```python
from build123d import *

# Parameters (mm, degrees)
SKETCH1_R           = 50
SKETCH1_W           = 25.4
SKETCH1_H           = 25.4
BOSS_EXTRUDE1_DEPTH = 5


with BuildPart() as part:
    # Sketch1 → Boss-Extrude1 (new body)
    with BuildSketch(Plane(origin=(0, 0, 0), x_dir=(1, 0, 0), z_dir=(0, 1, 0))):
        with BuildLine():
            Line((175.4, 110), (201.990098767, 110))
            ThreePointArc((201.990098767, 110), (230, 0), (201.990098767, -110))
            Line((201.990098767, -110), (175.4, -110))
            Line((175.4, -110), (175.4, -115))
            Line((175.4, -115), (199.18584287, -115))
            ThreePointArc((199.18584287, -115), (162.634559673, -162.634559673), (115, -199.18584287))
            Line((115, -199.18584287), (115, -175.4))
            Line((115, -175.4), (110, -175.4))
            Line((110, -175.4), (110, -201.990098767))
            ThreePointArc((110, -201.990098767), (0, -230), (-110, -201.990098767))
            Line((-110, -201.990098767), (-110, -175.4))
            Line((-110, -175.4), (-115, -175.4))
            Line((-115, -175.4), (-115, -199.18584287))
            ThreePointArc((-115, -199.18584287), (-162.634559673, -162.634559673), (-199.18584287, -115))
            Line((-199.18584287, -115), (-175.4, -115))
            Line((-175.4, -115), (-175.4, -110))
            Line((-175.4, -110), (-201.990098767, -110))
            ThreePointArc((-201.990098767, -110), (-230, 0), (-201.990098767, 110))
            Line((-201.990098767, 110), (-175.4, 110))
            Line((-175.4, 110), (-175.4, 115))
            Line((-175.4, 115), (-199.18584287, 115))
            ThreePointArc((-199.18584287, 115), (-162.634559673, 162.634559673), (-115, 199.18584287))
            Line((-115, 199.18584287), (-115, 175.4))
            Line((-115, 175.4), (-110, 175.4))
            Line((-110, 175.4), (-110, 201.990098767))
            ThreePointArc((-110, 201.990098767), (0, 230), (110, 201.990098767))
            Line((110, 201.990098767), (110, 175.4))
            Line((110, 175.4), (115, 175.4))
            Line((115, 175.4), (115, 199.18584287))
            ThreePointArc((115, 199.18584287), (162.634559673, 162.634559673), (199.18584287, 115))
            Line((199.18584287, 115), (175.4, 115))
            Line((175.4, 115), (175.4, 110))
        make_face()
        with Locations(Location((0, 0, 0), (0, 0, 270))):
            Circle(SKETCH1_R, mode=Mode.SUBTRACT)
        with Locations((127.7, 127.7)):
            Rectangle(SKETCH1_W, SKETCH1_H, mode=Mode.SUBTRACT)
        with Locations((-127.7, 127.7)):
            Rectangle(SKETCH1_W, SKETCH1_H, mode=Mode.SUBTRACT)
        with Locations((127.7, -127.7)):
            Rectangle(SKETCH1_W, SKETCH1_H, mode=Mode.SUBTRACT)
        with Locations((-127.7, -127.7)):
            Rectangle(SKETCH1_W, SKETCH1_H, mode=Mode.SUBTRACT)
        with BuildLine():
            Line((184.4, 26.5), (184.4, -26.5))
            ThreePointArc((184.4, -26.5), (183.374873734, -28.974873734), (180.9, -30))
            Line((180.9, -30), (179.9, -30))
            ThreePointArc((179.9, -30), (177.425126266, -28.974873734), (176.4, -26.5))
            Line((176.4, -26.5), (176.4, 26.5))
            ThreePointArc((176.4, 26.5), (177.425126266, 28.974873734), (179.9, 30))
            Line((179.9, 30), (180.9, 30))
            ThreePointArc((180.9, 30), (183.374873734, 28.974873734), (184.4, 26.5))
        make_face(mode=Mode.SUBTRACT)
        with BuildLine():
            Line((-26.5, 184.4), (26.5, 184.4))
            ThreePointArc((26.5, 184.4), (28.974873734, 183.374873734), (30, 180.9))
            Line((30, 180.9), (30, 179.9))
            ThreePointArc((30, 179.9), (28.974873734, 177.425126266), (26.5, 176.4))
            Line((26.5, 176.4), (-26.5, 176.4))
            ThreePointArc((-26.5, 176.4), (-28.974873734, 177.425126266), (-30, 179.9))
            Line((-30, 179.9), (-30, 180.9))
            ThreePointArc((-30, 180.9), (-28.974873734, 183.374873734), (-26.5, 184.4))
        make_face(mode=Mode.SUBTRACT)
        with BuildLine():
            Line((26.5, -184.4), (-26.5, -184.4))
            ThreePointArc((-26.5, -184.4), (-28.974873734, -183.374873734), (-30, -180.9))
            Line((-30, -180.9), (-30, -179.9))
            ThreePointArc((-30, -179.9), (-28.974873734, -177.425126266), (-26.5, -176.4))
            Line((-26.5, -176.4), (26.5, -176.4))
            ThreePointArc((26.5, -176.4), (28.974873734, -177.425126266), (30, -179.9))
            Line((30, -179.9), (30, -180.9))
            ThreePointArc((30, -180.9), (28.974873734, -183.374873734), (26.5, -184.4))
        make_face(mode=Mode.SUBTRACT)
        with BuildLine():
            Line((-184.4, -26.5), (-184.4, 26.5))
            ThreePointArc((-184.4, 26.5), (-183.374873734, 28.974873734), (-180.9, 30))
            Line((-180.9, 30), (-179.9, 30))
            ThreePointArc((-179.9, 30), (-177.425126266, 28.974873734), (-176.4, 26.5))
            Line((-176.4, 26.5), (-176.4, -26.5))
            ThreePointArc((-176.4, -26.5), (-177.425126266, -28.974873734), (-179.9, -30))
            Line((-179.9, -30), (-180.9, -30))
            ThreePointArc((-180.9, -30), (-183.374873734, -28.974873734), (-184.4, -26.5))
        make_face(mode=Mode.SUBTRACT)
    extrude(amount=BOSS_EXTRUDE1_DEPTH)


solid = part.part
```
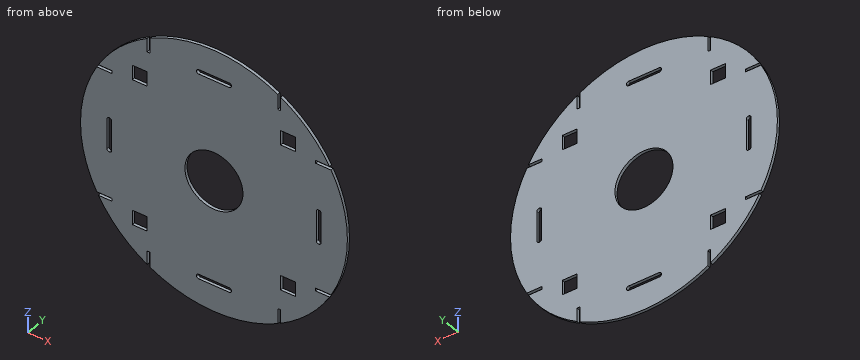
Input: part model. Units: mm. Frame: model coordinates. Give positions to 0.01 mm unless a question says otherwise; leave off trailing zeros. Write each loop counter-clockwise with the first axis right and the second up, starting at its lowest first coordinate (ties: lowest second). Pieces come first, ordered by that corner, then holes. Notation, with made-up numbers: (65.5, 73.5) - (109.5, 73.5) arc R24 cw to (109.5, 86.5) - close; hole circle Ø11 at (60.25, 73). An arc over 180 degrees is marked (long way). Write item = value, one per line. Start each with the question number.
1. Section query A-A, the plane z = 0. Output: boundary loops of the cut face in (x, y).
2. Section query C-C, the plane z = 135. Output: boundary loops of the cut face in (x, y).
3. First-contact query: pin 1 Ø2.5 at (y, z) = (2.5, 134) entering from -X; pin 2 Ø3 at (y, z) = (4.5, 98) entering from -X; pin 3 Ø2.5 at (x, y) = (-127.5, 3.5) entering from +Z. Flat tips, straight axial feed; report the tip coordinate or a pass-through.
4. Ray query, L1, parallel to X at y = 4.55, z = -18; L2, parallel to X at y = 2.8, z = 121.5; L3, parallel to Z at x = 123.5, y = 0.8. Return the intervals inside material, ascending.
5. Section query D-D, the plane y = 2.2. Count the separate pieces of the cut face and the enclosed holes in it, then the cut area to 3 significant figures.
6. Section query B-B, the plane x = 0. Output: boundary loops of the cut face in (y, z).
Check sheet entries:
q1.outline = (-230, 0) - (-184.4, 0) - (-184.4, 5) - (-230, 5) - close; (-176.4, 0) - (-50, 0) - (-50, 5) - (-176.4, 5) - close; (50, 0) - (176.4, 0) - (176.4, 5) - (50, 5) - close; (184.4, 0) - (230, 0) - (230, 5) - (184.4, 5) - close
q2.outline = (-186.21, 0) - (-140.4, 0) - (-140.4, 5) - (-186.21, 5) - close; (-115, 0) - (115, 0) - (115, 5) - (-115, 5) - close; (140.4, 0) - (186.21, 0) - (186.21, 5) - (140.4, 5) - close
q3.pin_1 = -187.82
q3.pin_2 = -208.78
q3.pin_3 = 192.25
q4.L1 = -229.29 to -184.4, -176.4 to -46.65, 46.65 to 176.4, 184.4 to 229.29
q4.L2 = -195.29 to -140.4, -115 to 115, 140.4 to 195.29
q4.L3 = -194.03 to -140.4, -115 to 115, 140.4 to 194.03
q5.separate_pieces = 1
q5.enclosed_holes = 9
q5.area = 153,000 mm2
q6.outline = (0, -230) - (5, -230) - (5, -184.4) - (0, -184.4) - close; (0, -176.4) - (5, -176.4) - (5, -50) - (0, -50) - close; (0, 50) - (5, 50) - (5, 176.4) - (0, 176.4) - close; (0, 184.4) - (5, 184.4) - (5, 230) - (0, 230) - close
